Geometry check sheet. Reference: drawing and pictorial views, mm from the part's lowest x, y, z. Give positions to 0.01 mm unless a question says otherwise; leave off trailing zeros. Write each loop counter-clockwise with the first axis right and the second up, starting at its lowest first coordinate (ties: lowest second). Pieces come first, ordered by that corner, then holes. Notation, with made-up numbers: M 45,2 L 91,2 A17 cw 91,17 Z; hole C 23,12 d10. An arc over 180 degrees is marked long. One line per item, written item: value. Start each with the question number.
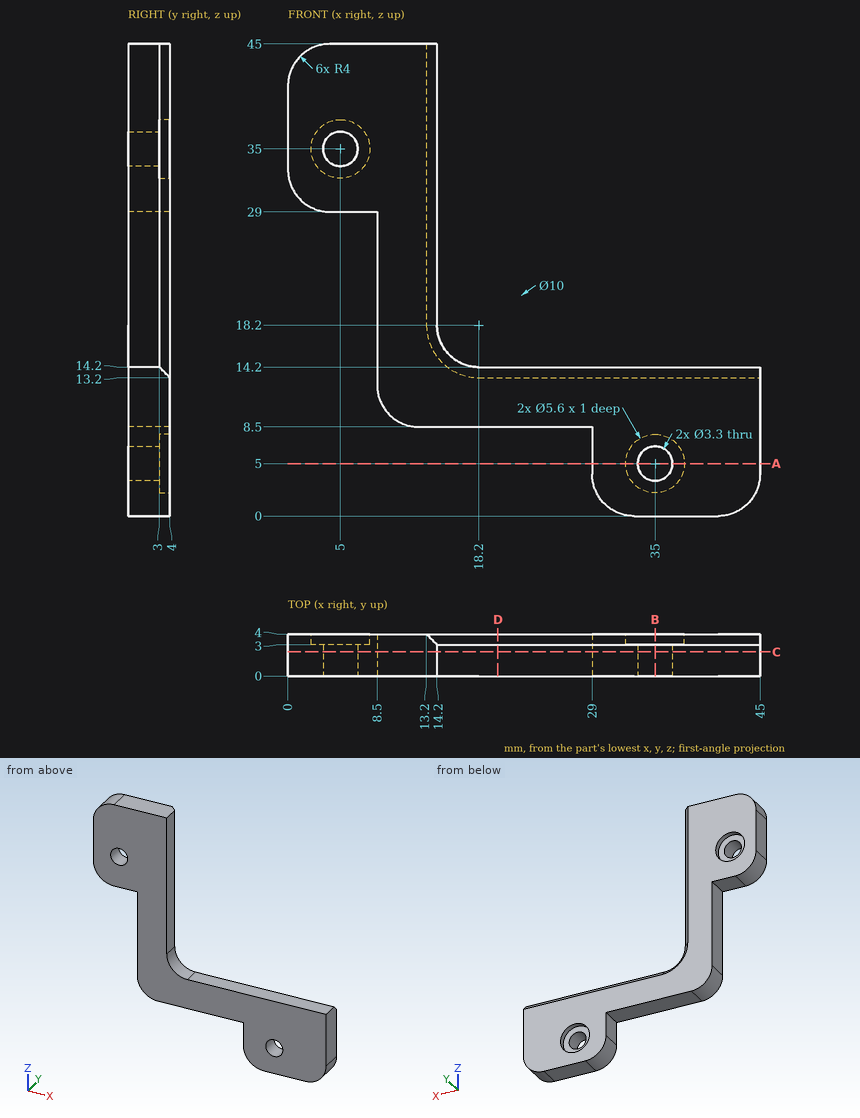
1) Cross-section at D-D (x = 20). Record the boundary of the cut face in (y, z).
2) Material ranges on L1, parallel to X at y = 1.1, z = 5; L2, parallel to Z at x = 35, y = 2.1; L3, parallel to X at y = 3.3, z = 5, recorded low to high. Write a range as from..to.
3) Cross-section at B-B (x = 35). Record the boundary of the cut face in (y, z).
4) Cross-section at C-C (y = 2.3). Record the boundary of the cut face in (x, z), plus the area to 3 significant figures.
5) Gauge pin test, flat ends, axial feed: pin 1 (0.9 mm diameter, centred on y = 2, z = 35, fed in from +X); pin 2 (2 mm diameter, centred on y = 1.5, z = 24, fed in from -X); pin 3 (5 mm diameter, centred on x = 35, z = 5, fed in from +Y). Record the tip position at first contact, or that the pin passes through.
6) Cross-section at A-A (z = 5). Record the boundary of the cut face in (x, y).
Data:
1. outline: M 0,8.5 L 4,8.5 L 4,13.2 L 3,14.2 L 0,14.2 Z
2. L1: x = 29..33.35, 36.65..45
2. L2: z = 0..3.35, 6.65..14.2
2. L3: x = 29..32.2, 37.8..45
3. outline: M 0,0 L 4,0 L 4,2.2 L 3,2.2 L 3,3.35 L 0,3.35 Z; M 0,6.65 L 3,6.65 L 3,7.8 L 4,7.8 L 4,13.2 L 3,14.2 L 0,14.2 Z
4. outline: M 0,33 A4 ccw 4,29 L 8.5,29 L 8.5,12.5 A4 ccw 12.5,8.5 L 29,8.5 L 29,4 A4 ccw 33,0 L 41,0 A4 ccw 45,4 L 45,14.2 L 18.2,14.2 A4 cw 14.2,18.2 L 14.2,45 L 4,45 A4 ccw 0,41 Z; hole C 5,35 d3.3; hole C 35,5 d3.3
4. area: 625 mm2
5. pin 1: stops at x = 14.2
5. pin 2: stops at x = 8.5
5. pin 3: stops at y = 3
6. outline: M 29,0 L 33.35,0 L 33.35,3 L 32.2,3 L 32.2,4 L 29,4 Z; M 36.65,0 L 45,0 L 45,4 L 37.8,4 L 37.8,3 L 36.65,3 Z
